Print and shaded views of the part. All mm, measured from the part's lowest x, y and z. A direction names the side the tool comes from. Round coordinates to 2 decimals unless told otherwise and drop trailing zeros. Write each loop counter-clockwise with the first axis right and the second up, starting at its lowest first coordinate (ties: lowest second). Pieces come first, ordered by that corner, then holes. Notation, with made-up numbers: M 12.5,12 L 51.5,12 A11 cw 51.5,16 Z; hole C 75.25,72 d9. An arc over 180 degrees is marked long. Write item = value, one per line. Start each with the question number.
Q1. Tool access for the marked faces 1, 2 and 3: list every direction of +Z, -Z, +X, -X, +Y, -Y with a clear straight run to the whole face (end or side of a thin tool).
Q2. Band-saw the part on D-D on z = 10.5. Write the cut outline in (x, y).
Q3. Pull direction Z, two halves, no side cores. Call the marked faces 4, 5 and 6: released by +Z, released by -Z, zero draft, split by the parting line, or undercut.
Q4. Band-saw the part on C-C on z = 7. Write the cut outline in (x, y).
Q5. Probe L1, parallel to X at y = 5.25, z = 7; L2, parallel to X at y = 31.5, z = 2; L3, parallel to Z at x = 37.05, y = 2.5. List the from-to ranges inside material, lowest first.
Q6. Band-saw the part on B-B on x = 37.05. Write the cut outline in (y, z), plus the area to 4 significant figures.
Q7. Drop flat-ended pins along their axis: P1, Ø5.5, axis at x = 39, z = 7.5, coming from the +Y side; P2, Ø1, axis at y = 21, z = 11.5, coming from the -X side; P3, Ø3, axis at y = 23.5, z = 7, coming from the +X side. Give the stop position or say it passes through.
Q8. Band-saw the part on A-A on y = 23. Write the cut outline in (x, z).
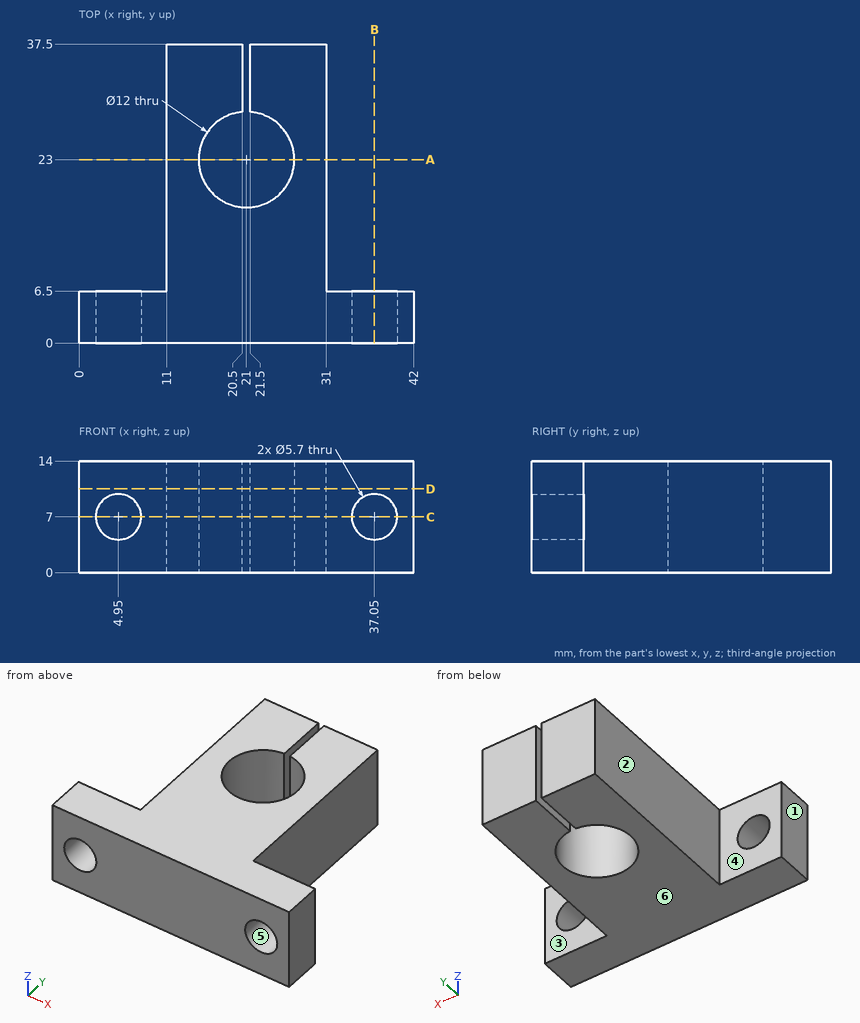
Conclusion:
q1.face_1 = +Z, -Z, -X, +Y, -Y
q1.face_2 = +Z, -Z, -X, +Y
q1.face_3 = +Z, -Z, +X, +Y
q2.outline = M 0,0 L 42,0 L 42,6.5 L 31,6.5 L 31,37.5 L 21.5,37.5 L 21.5,28.98 A6 cw long 20.5,28.98 L 20.5,37.5 L 11,37.5 L 11,6.5 L 0,6.5 Z
q3.face_4 = zero draft
q3.face_5 = undercut
q3.face_6 = released by -Z
q4.outline = M 0,0 L 2.1,0 L 2.1,6.5 L 0,6.5 Z; M 7.8,0 L 34.2,0 L 34.2,6.5 L 31,6.5 L 31,37.5 L 21.5,37.5 L 21.5,28.98 A6 cw long 20.5,28.98 L 20.5,37.5 L 11,37.5 L 11,6.5 L 7.8,6.5 Z; M 39.9,0 L 42,0 L 42,6.5 L 39.9,6.5 Z
q5.L1 = 0 to 2.1, 7.8 to 34.2, 39.9 to 42
q5.L2 = 11 to 20.5, 21.5 to 31
q5.L3 = 0 to 4.15, 9.85 to 14
q6.outline = M 0,0 L 6.5,0 L 6.5,4.15 L 0,4.15 Z; M 0,9.85 L 6.5,9.85 L 6.5,14 L 0,14 Z
q6.area = 53.95 mm^2
q7.P1 = 6.5
q7.P2 = 11
q7.P3 = 31
q8.outline = M 11,0 L 15,0 L 15,14 L 11,14 Z; M 27,0 L 31,0 L 31,14 L 27,14 Z
